Autodesk Fusion 360 part; units mm, degrees
sketch "Sketch1" plane through (0, 0, 0) normal (0, 1, 0) x (1, 0, 0)
  circle A0 centre (0, 0) radius 6.5
  circle A1 centre (0, 7.5) radius 18.375
  line L0 (0, 0) -> (0, 7.5)
  circle A2 centre (0, 7.5) radius 15.5 construction
  line L1 (-26.0681, 7.5) -> (26.0681, 7.5) construction
  circle A3 centre (15.5, 7.5) radius 1.5
  circle A4 centre (7.75, 20.9234) radius 1.5
  circle A5 centre (-7.75, 20.9234) radius 1.5
  circle A6 centre (-15.5, 7.5) radius 1.5
  circle A7 centre (-7.75, -5.9234) radius 1.5
  circle A8 centre (7.75, -5.9234) radius 1.5
  line L2 (-19.977, -10.875) -> (20.9733, -10.875) construction
  dimension "d1" = 13
  dimension "d2" = 36.75
  dimension "d3" = 7.5
  dimension "d4" = 31
  dimension "d5" = 3
  dimension "d7" = 360
  dimension "d10" = 10.875
extrude "Extrude1" add sketch "Sketch1" along normal blind 0.6
CAD build for the part. Positions are in the model's coordinates, mm. Round coordinates to 2 decimals unless told otherwise and drop trailing zeros. Write each loop counter-clockwise with the first axis right and the second up, starting at its lowest first coordinate (ties: lowest second). Pieces come first, ordered by that corner, then holes. Notation, with made-up numbers: (11, 72.25) - (52, 72.25) arc R18 cw to (52, 100.25) - close; hole circle Ø11 at (10.25, 20). An arc over 180 degrees is marked (long way). Return JSON: item names as keys, results as strings. Group by question number.
Item 1: Mould opens along X. For faces 1 (the face through (0, 0.6, -8)), 2 (the face through (-16.7, 0.3, -8.4)), 3 (the face through (-5.158, 0.296, -3.955)), 4 (the face through (17.526, 0.296, -1.981)) say: +X half, -X half, draft (parallel to the pull), parting line (faces both ways), or undercut.
Item 2: Band-saw the part on A-A on z = -7.5. List the corners of the cut face in (x, y) (3 decimals).
Item 3: Probe probe 1 along X at (y, z) = (0.25, -7.5) (3 decimals); probe 2 along Z at (x, y) = (0, 0.3) (3 decimals); probe 3 along Z at (x, y) = (-7.75, 0.15). List the from-to ranges inside material, lowest first.
Item 4: Band-saw the part on B-B on x = 0. List the corners of the cut face in (y, z) (3 decimals), plus the area to 4 significant figures.
Item 5: Band-saw the part on C-C on z = 0. List the corners of the cut face in (x, y).
Item 6: Band-saw the part on D-D on y = 0.5. List the corners of the cut face in (x, z) (3 decimals).
Item 7: Flat gauge pin, fed straight in: pin 1 Ø8 at (x, z) = (0, 0) entering from -Y. Where does the tip first touch, or does it go through?
Resolved:
{
 "1": {"face 1": "draft", "face 2": "undercut", "face 3": "undercut", "face 4": "parting line"},
 "2": {"outline": "(-18.375, 0) - (-17, 0) - (-17, 0.6) - (-18.375, 0.6) - close; (-14, 0) - (14, 0) - (14, 0.6) - (-14, 0.6) - close; (17, 0) - (18.375, 0) - (18.375, 0.6) - (17, 0.6) - close"},
 "3": {"probe 1": "x = -18.375 to -17, -14 to 14, 17 to 18.375", "probe 2": "z = -25.875 to -6.5, 6.5 to 10.875", "probe 3": "z = -24.16 to -22.42, -19.42 to 4.42, 7.42 to 9.16"},
 "4": {"outline": "(0, -25.875) - (0.6, -25.875) - (0.6, -6.5) - (0, -6.5) - close; (0, 6.5) - (0.6, 6.5) - (0.6, 10.875) - (0, 10.875) - close", "area": "14.25 mm²"},
 "5": {"outline": "(-16.77, 0) - (-6.5, 0) - (-6.5, 0.6) - (-16.77, 0.6) - close; (6.5, 0) - (16.77, 0) - (16.77, 0.6) - (6.5, 0.6) - close"},
 "6": {"outline": "circle Ø36.75 at (0, -7.5); hole circle Ø3 at (-15.5, -7.5); hole circle Ø3 at (-7.75, -20.923); hole circle Ø3 at (-7.75, 5.923); hole circle Ø13 at (0, 0); hole circle Ø3 at (7.75, -20.923); hole circle Ø3 at (7.75, 5.923); hole circle Ø3 at (15.5, -7.5)"},
 "7": {"pin 1": "passes through"}
}
